Here's how the part is built. I have some questions about the finished solid (model axes, mm). A direction names the side the tool comes from. Coordinates: 2 decimals unless noted, no trailing zeros. Order: outer loops, then holes, each group sorted by start corner. A loop starts at its lowest first (then second) coordinate and runs counter-clockwise, first axis right, second up. Notation, with made-up numbers: (31, 48) -> (75, 48) arc R14 ccw to (75, 72) -> close; hole circle Ø5 at (80, -32). An arc over 180 degrees is marked (long way). One line per item, written item: value. Start each with the question number.
```python
from build123d import *

# Parameters (mm, degrees)
EXTRUDE_1_DEPTH = 3
EXTRUDE_2_DEPTH = 3


with BuildPart() as part:
    # 草图1 → 凸台-拉伸1 (new body)
    with BuildSketch(Plane.XY):
        with BuildLine():
            ThreePointArc((-17.306693672, 14.907284768), (-26.806693672, 24.407284768), (-36.306693672, 14.907284768))
            ThreePointArc((-36.306693672, 14.907284768), (-34.403568029, 9.203119623), (-29.456693672, 5.784374048))
            Line((-29.456693672, 5.784374048), (-29.456693672, 11.757284768))
            ThreePointArc((-29.456693672, 11.757284768), (-26.806693672, 14.407284768), (-24.156693672, 11.757284768))
            Line((-24.156693672, 11.757284768), (-24.156693672, 5.784374048))
            ThreePointArc((-24.156693672, 5.784374048), (-19.209819315, 9.203119623), (-17.306693672, 14.907284768))
        make_face()
        with BuildLine():
            ThreePointArc((-29.456693672, 5.784374048), (-34.403568029, 9.203119623), (-36.306693672, 14.907284768))
            Line((-36.306693672, 14.907284768), (-36.306693672, -23.592715232))
            Line((-36.306693672, -23.592715232), (-29.456693672, -23.592715232))
            Line((-29.456693672, -23.592715232), (-29.456693672, 5.784374048))
        make_face()
        with BuildLine():
            Line((-17.306693672, -23.592715232), (-17.306693672, 14.907284768))
            ThreePointArc((-17.306693672, 14.907284768), (-19.209819315, 9.203119623), (-24.156693672, 5.784374048))
            Line((-24.156693672, 5.784374048), (-24.156693672, -23.592715232))
            Line((-24.156693672, -23.592715232), (-17.306693672, -23.592715232))
        make_face()
    extrude(amount=-EXTRUDE_1_DEPTH)

    # 草图2 → 凸台-拉伸2 (add)
    with BuildSketch(Plane.XZ.offset(23.592715232)):
        with BuildLine():
            ThreePointArc((-34.81143952, 41.116057458), (-35.925221118, 38.665043569), (-36.306693672, 36))
            ThreePointArc((-36.306693672, 36), (-34.403568029, 30.295834855), (-29.456693672, 26.87708928))
            Line((-29.456693672, 26.87708928), (-29.456693672, 32.85))
            ThreePointArc((-29.456693672, 32.85), (-26.806693672, 35.5), (-24.156693672, 32.85))
            Line((-24.156693672, 32.85), (-24.156693672, 26.87708928))
            ThreePointArc((-24.156693672, 26.87708928), (-19.209819315, 30.295834855), (-17.306693672, 36))
            ThreePointArc((-17.306693672, 36), (-17.688166227, 38.665043569), (-18.801947824, 41.116057458))
            Line((-18.801947824, 41.116057458), (-34.81143952, 41.116057458))
        make_face()
        with BuildLine():
            ThreePointArc((-18.801947824, 41.116057458), (-26.806693672, 45.5), (-34.81143952, 41.116057458))
            Line((-34.81143952, 41.116057458), (-18.801947824, 41.116057458))
        make_face()
        with BuildLine():
            Line((-36.306693672, 36), (-36.306693672, 0))
            Line((-36.306693672, 0), (-29.456693672, 0))
            Line((-29.456693672, 0), (-29.456693672, 26.87708928))
            ThreePointArc((-29.456693672, 26.87708928), (-34.403568029, 30.295834855), (-36.306693672, 36))
        make_face()
        with BuildLine():
            Line((-24.156693672, 26.87708928), (-24.156693672, -3))
            Line((-24.156693672, -3), (-17.306693672, -3))
            Line((-17.306693672, -3), (-17.306693672, 36))
            ThreePointArc((-17.306693672, 36), (-19.209819315, 30.295834855), (-24.156693672, 26.87708928))
        make_face()
    extrude(amount=-EXTRUDE_2_DEPTH)


solid = part.part
```
Q1. Imagine slicing it at B-B (z = 20.5). Write out the boundary of the cut face in (x, y).
Q2. Imagine slicing it at A-A (y = 6.5). Write out the boundary of the cut face in (x, z).
Q3. I need wall thicknesses on line 1 (X direction, y = -21, z = 9.5); line 2 (Z direction, x = -20.75, y = 13); line 3 (Y direction, x = -23, z = 19). Which ranges of each line are inside material? Lowest first, please.
Q4. If we mould it in two halves opening along X, with no side actions, what happens to faces 1 (the face through (-31, 2, 0)), 2 (the face through (-24.157, -22, 7)), 3 (the face through (-17.307, -13, -1))? For each: +X half, -X half, draft (parallel to the pull), parting line (faces both ways), or undercut.
Q5. For faces 4 (the face through (-26.865, 14.407, -1.479)), 5 (the face through (-29.457, -14, -1)), 6 (the face through (-31, -20.593, 23)), which set-ups out of +Z, -Z, +X, -X, +Y, -Y let a thin tool reach every point of the face, with its end or its side?
Q6. For P1, Ø5.5, axis at x = -28.5, y = -6, coming from the +Z side; P2, Ø3, axis at x = -22, z = 27, coming from the +Y side, each with a flat end and sliding along its axis, tell me the tip position at first contact or that it passes through.
Completed:
1. outline: (-36.31, -23.59) -> (-29.46, -23.59) -> (-29.46, -20.59) -> (-36.31, -20.59) -> close; (-24.16, -23.59) -> (-17.31, -23.59) -> (-17.31, -20.59) -> (-24.16, -20.59) -> close
2. outline: (-36.31, -3) -> (-29.46, -3) -> (-29.46, 0) -> (-36.31, 0) -> close; (-24.16, -3) -> (-17.31, -3) -> (-17.31, 0) -> (-24.16, 0) -> close
3. line 1: x = -36.31 to -29.46, -24.16 to -17.31
3. line 2: z = -3 to 0
3. line 3: y = -23.59 to -20.59
4. face 1: draft
4. face 2: undercut
4. face 3: +X half
5. face 4: +Z, -Z, -Y
5. face 5: -Z, -Y
5. face 6: +Z, +X, -X, +Y
6. P1: stops at z = 0
6. P2: stops at y = -20.59
